```python
from build123d import *

# Parameters (mm, degrees)
SKETCH1_W           = 6.731
SKETCH1_H           = 6.731
BOSS_EXTRUDE1_DEPTH = 36.5125
FILLET1_R           = 0.396875
FILLET2_R           = 1.5875


with BuildPart() as part:
    # Sketch1 → Boss-Extrude1 (new body)
    with BuildSketch(Plane.XY):
        Polygon((4.949335183, -2.8575), (4.949335183, 2.8575), (0, 5.715), (-4.949335183, 2.8575), (-4.949335183, -2.8575), (0, -5.715), align=None)
        Rectangle(SKETCH1_W, SKETCH1_H, mode=Mode.SUBTRACT)
    extrude(amount=BOSS_EXTRUDE1_DEPTH)

    # Fillet1
    fillet1_edges = [part.edges().sort_by_distance(p)[0] for p in [
        (3.3655, 0, 0),
        (3.3655, -3.3655, 18.25625),
        (0, 3.3655, 0),
        (3.3655, 3.3655, 18.25625),
        (-3.3655, 0, 0),
        (-3.3655, 3.3655, 18.25625),
        (0, -3.3655, 0),
        (-3.3655, -3.3655, 18.25625),
        (3.3655, 0, 36.5125),
        (0, 3.3655, 36.5125),
        (-3.3655, 0, 36.5125),
        (0, -3.3655, 36.5125),
    ]]
    fillet(fillet1_edges, radius=FILLET1_R)

    # Fillet2
    fillet2_edges = [part.edges().sort_by_distance(p)[0] for p in [
        (0, -5.715, 18.25625),
        (-4.949335183, -2.8575, 18.25625),
        (-4.949335183, 2.8575, 18.25625),
        (0, 5.715, 18.25625),
        (4.949335183, 2.8575, 18.25625),
        (4.949335183, -2.8575, 18.25625),
    ]]
    fillet(fillet2_edges, radius=FILLET2_R)


solid = part.part
```
Can you work these out from the model? Positions are in its coordinate system, mm. A direction names the side the tool comes from. Give positions to 0.01 mm unless a question says otherwise; leave off trailing zeros. Loops run counter-clockwise (first coordinate to the right, second up) from the corner with the lowest first, then second, coordinate; pieces in that order, holes last. Notation, with made-up numbers: M 74,7 L 123,7 A20 ccw 123,22 Z; hole C 51.5,39.25 d8. An arc over 180 degrees is marked long. One line per question, with ' | ' between items. Start each with the question number.
Q1. For pin 1 Ø2 at (x, z) = (-1.5, 7.5) entering from +Y; pin 2 Ø1 at (y, z) = (3.5, 28.5) entering from -X; pin 3 Ø4 at (x, y) = (-2.5, 3.5) entering from +Z, each with a flat end and sliding along its axis, tell me the tip position at first contact or that it passes through.
Q2. For faces 5 (the flat face through (0, 3.366, 18)), 6 (the cylindrical face through (4.742, -2.725, 18.512)), which set-ups out of +Z, -Z, +X, -X, +Y, -Y let a thin tool reach every point of the face, with its end or its side?
Q3. If I drill on line 1 (X direction, y = 1, z = 16.5); line 2 (Y direction, x = -1, z = 20.5); line 3 (Y direction, x = -0.5, z = 5.5), over which ranges is the centre line in solid material (lowest first)? Write a range as from..to.
Q4. If we section it at D-D (y = 4.25): Please give me the cut outline in (x, z).
Q5. If we section it at B-B (z = 19): Please give me the cut outline in (x, y) (1 decimal), plus the area to 3 significant figures.
Q6. If we section it at C-C (x = -2): Please give me the cut outline in (y, z).
Q7. If we mould it in two halves opening along Y, with no side actions, what happens to faces 1 (the flat face through (0, -4, 36.512)), 2 (the cylindrical face through (-4.731, -2.745, 18.512)), 3 (the flat face through (-3.366, 0, 18)), 4 (the flat face through (2.5, 4.27, 18))? For each: +Y half, -Y half, draft (parallel to the pull), parting line (faces both ways), or undercut.
Q8. If we section it at A-A (y = 0.5): Please give me the cut outline in (x, z).
Computed:
1) pin 1: stops at y = 5.39 | pin 2: stops at x = -4.54 | pin 3: stops at z = 36.51
2) face 5: +Z, -Z | face 6: +Z, -Z, +X, -Y
3) line 1: x = -4.95..-3.37, 3.37..4.95 | line 2: y = -5.14..-3.37, 3.37..5.14 | line 3: y = -5.39..-3.37, 3.37..5.39
4) outline: M -2.54,0 L 2.54,0 L 2.54,36.51 L -2.54,36.51 Z
5) outline: M -4.9,-1.9 A1.6 ccw -4.2,-3.3 L -0.8,-5.3 A1.6 ccw 0.8,-5.3 L 4.2,-3.3 A1.6 ccw 4.9,-1.9 L 4.9,1.9 A1.6 ccw 4.2,3.3 L 0.8,5.3 A1.6 ccw -0.8,5.3 L -4.2,3.3 A1.6 ccw -4.9,1.9 Z; hole M -3.4,-3 A0.4 ccw -3,-3.4 L 3,-3.4 A0.4 ccw 3.4,-3 L 3.4,3 A0.4 ccw 3,3.4 L -3,3.4 A0.4 ccw -3.4,3 Z | area: 38.9 mm²
6) outline: M -4.56,0 L -3.76,0 A0.4 ccw -3.37,0.4 L -3.37,36.12 A0.4 ccw -3.76,36.51 L -4.56,36.51 Z; M 3.37,0.4 A0.4 ccw 3.76,0 L 4.56,0 L 4.56,36.51 L 3.76,36.51 A0.4 ccw 3.37,36.12 Z
7) face 1: draft | face 2: -Y half | face 3: undercut | face 4: +Y half
8) outline: M -4.95,0 L -3.76,0 A0.4 ccw -3.37,0.4 L -3.37,36.12 A0.4 ccw -3.76,36.51 L -4.95,36.51 Z; M 3.37,0.4 A0.4 ccw 3.76,0 L 4.95,0 L 4.95,36.51 L 3.76,36.51 A0.4 ccw 3.37,36.12 Z
